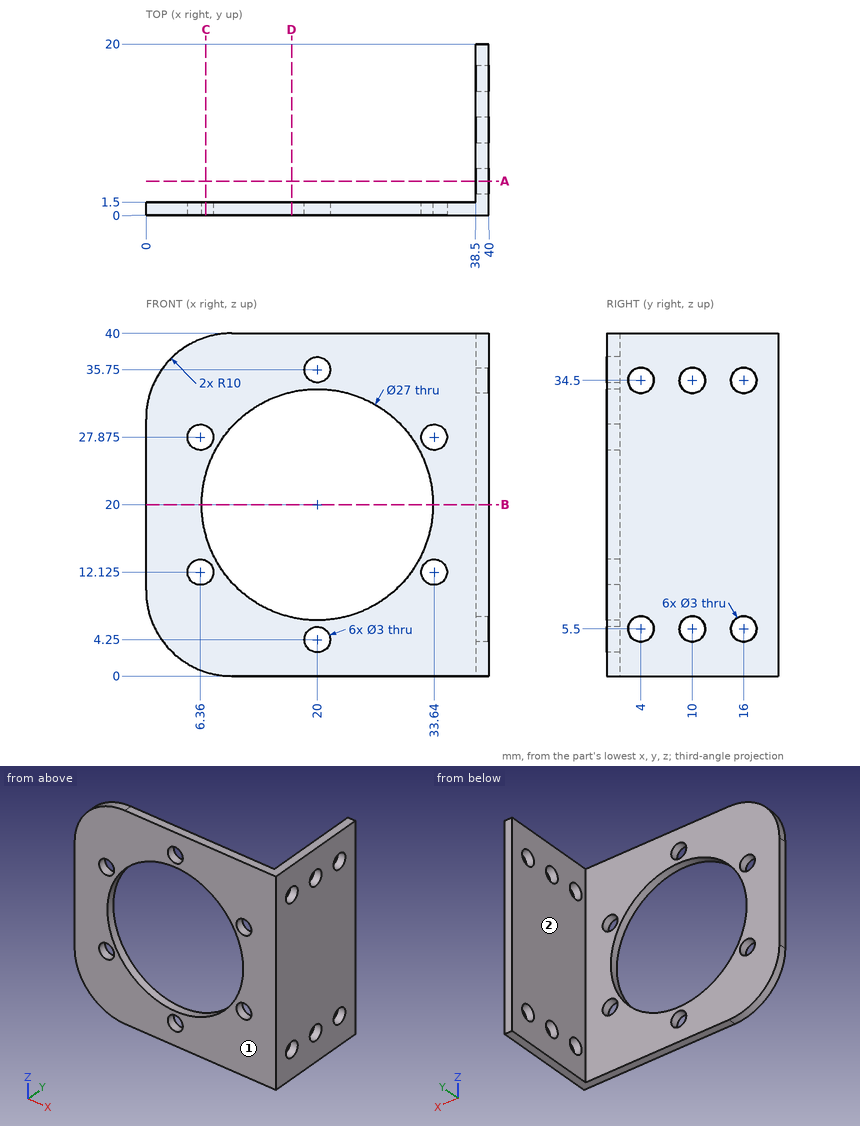
Design review of the part shown in the three views and the two pictorial views. Dimensions are in mm from the part's minimum x, y and z. A direction names the side the tool comes from. Give positions to 0.01 mm unless a question says otherwise; leave off trailing zeros. Write each loop counter-clockwise with the first axis right and the second up, starting at its lowest first coordinate (ties: lowest second). Pieces come first, ordered by that corner, then holes. Notation, with made-up numbers: M 87,14.25 L 100,14.25 A35 ccw 100,53.25 Z; hole C 50.25,-33 d4. An arc over 180 degrees is marked long. One line per item, written item: value.
1) For P1, Ø11.5, axis at x = 24.5, z = 16.5, coming from the +Y side; P2, Ø4, axis at x = 19, y = 3, coming from the -Z side; P3, Ø4, axis at x = 33.5, z = 5, coming from the +Y side; P4, Ø12, axis at y = 16.5, z = 9.5, coming from the -X side, all flat-tipped, find the tip position at first contact; note any pin that passes through.
Results are:
P1: passes through
P2: stops at z = 0
P3: stops at y = 1.5
P4: stops at x = 38.5
2) For line 1 (Y direction, x = 38.9, z = 34.5); line 2 (Z direction, x = 38.9, y = 10); line 3 (Y direction, x = 39, z = 5), list the stretches that pass through material, from the lowest coordinate up. Write a range as from..to.
Results are:
line 1: y = 0..2.5, 5.5..8.5, 11.5..14.5, 17.5..20
line 2: z = 0..4, 7..33, 36..40
line 3: y = 0..2.59, 5.41..8.59, 11.41..14.59, 17.41..20
3) Take a section at C-C, the plane x = 7. Write out the cut boundary in (y, z).
Results are:
outline: M 0,0.46 L 1.5,0.46 L 1.5,10.77 L 0,10.77 Z; M 0,13.48 L 1.5,13.48 L 1.5,16.36 L 0,16.36 Z; M 0,23.64 L 1.5,23.64 L 1.5,26.52 L 0,26.52 Z; M 0,29.23 L 1.5,29.23 L 1.5,39.54 L 0,39.54 Z
4) Take a section at B-B, the plane z = 20. Write out the cut boundary in (x, y).
Results are:
outline: M 0,0 L 6.5,0 L 6.5,1.5 L 0,1.5 Z; M 33.5,0 L 40,0 L 40,20 L 38.5,20 L 38.5,1.5 L 33.5,1.5 Z
5) Take a section at A-A, the plane y = 4. Write out the cut boundary in (x, z).
Results are:
outline: M 38.5,0 L 40,0 L 40,4 L 38.5,4 Z; M 38.5,7 L 40,7 L 40,33 L 38.5,33 Z; M 38.5,36 L 40,36 L 40,40 L 38.5,40 Z
6) For the marked faces 1 and 2, list the 3-axis set-ups (+Z, -Z, +X, -X, +Y, -Y) from which the entire face can be reached by the end or side of a thin tool; tool diameter is ignored.
Results are:
face 1: +Z, -Z, +X, -X, -Y
face 2: +Z, -Z, -X, +Y
7) Take a section at D-D, the plane x = 17. Write out the cut boundary in (y, z), then the cut area to 3 significant figures.
Results are:
outline: M 0,0 L 1.5,0 L 1.5,6.84 L 0,6.84 Z; M 0,33.16 L 1.5,33.16 L 1.5,40 L 0,40 Z
area: 20.5 mm²
